```python
from build123d import *

# Parameters (mm, degrees)
SKETCH1_W           = 20.5
SKETCH1_H           = 21.3
BOSS_EXTRUDE1_DEPTH = 13.9
SKETCH2_R           = 6.221989568
BOSS_EXTRUDE2_DEPTH = 10.9


with BuildPart() as part:
    # Sketch1 → Boss-Extrude1 (new body)
    with BuildSketch(Plane(origin=(0, 0, 0), x_dir=(1, 0, 0), z_dir=(0, 1, 0))):
        Rectangle(SKETCH1_W, SKETCH1_H)
    extrude(amount=BOSS_EXTRUDE1_DEPTH)

    # Sketch2 → Boss-Extrude2 (add)
    with BuildSketch(Plane.XY.offset(10.65)):
        with Locations((-3.349791779, 7.996227622)):
            Circle(SKETCH2_R)
    extrude(amount=BOSS_EXTRUDE2_DEPTH)


solid = part.part
```
Build history of the part. All positions in model axes, mm. A direction names the side the tool comes from. Round coordinates to 2 decimals unless told otherwise and drop trailing zeros. Write each loop counter-clockwise with the first axis right and the second up, starting at its lowest first coordinate (ties: lowest second). Pieces come first, ordered by that corner, then holes. Notation, with made-up numbers: (46.25, -26.5) - (92.25, -26.5) arc R26 cw to (92.25, -3.5) - close; hole circle Ø4 at (-18, -14). An arc over 180 degrees is marked (long way). Answer as CSV lines item,"result".
Q1. Tool access for faces 1 (the flat face through (0, 13.9, 0)), 2 (the flat face through (0, 7, -10.65)), 3 (the cylindrical face through (-4.699, 1.922, 16.024)): list every direction of +Z, -Z, +X, -X, +Y, -Y with a clear straight run to the whole face (end or side of a thin tool).
Report:
face 1,"-Z, +X, -X, +Y"
face 2,"-Z, +X, -X, +Y, -Y"
face 3,"+Z"
Q2. Cut at A-A (y = 7). Write the cut outline in (x, z), and give its area (3 significant figures).
Report:
outline,"(-10.25, -10.65) - (10.25, -10.65) - (10.25, 10.65) - (2.79, 10.65) - (2.79, 21.55) - (-9.49, 21.55) - (-9.49, 10.65) - (-10.25, 10.65) - close"
area,"571 mm^2"
Q3. Drop a flat-ended pin along its axis: pin 1 (10 mm diameter, centred on x = -3.5, z = 1, fed in from +Y). Give the stop position or say it passes through.
Report:
pin 1,"stops at y = 13.9"
Q4. Cut at D-D (y = 13.25). Write the cut outline in (x, z).
Report:
outline,"(-10.25, -10.65) - (10.25, -10.65) - (10.25, 10.65) - (-0.02, 10.65) - (-0.02, 21.55) - (-6.68, 21.55) - (-6.68, 10.65) - (-10.25, 10.65) - close"
Q5. Cut at B-B (x = 5.25). Write the cut outline in (y, z).
Report:
outline,"(0, -10.65) - (13.9, -10.65) - (13.9, 10.65) - (0, 10.65) - close"
Q6. Cut at C-C (z = 9). Write the cut outline in (x, y).
Report:
outline,"(-10.25, 0) - (10.25, 0) - (10.25, 13.9) - (-10.25, 13.9) - close"
Q7. Drill centre lines: probe 1 along Z at (x, y) = (6.5, 3.5); probe 2 along Y at (x, z) = (-8.5, 5.5); probe 3 along Y at (x, z) = (-8, 17.5). Where is each one in solid material? Low to high. Write a range as [from, to].
Report:
probe 1,"z = [-10.65, 10.65]"
probe 2,"y = [0, 13.9]"
probe 3,"y = [3.86, 12.13]"
